Could you check a few things on this model? Use its own coordinates, in mm. Face numbers are marked on the shaded views. A direction names the side the tool comes from. Round coordinates to 2 decimals unless told otherwise and drop trailing zeros. Write each loop counter-clockwise with the first axis right and the second up, starting at its lowest first coordinate (ties: lowest second). Pieces come first, ordered by that corner, then holes. Notation, with made-up numbers: M -7,27.5 L 8,27.5 A19 ccw 8,38.5 Z; hole C -27.75,71.25 d10. An arc over 180 degrees is marked long. One line per item, written item: value. Start each with the question number.
(1) I want a section at B-B on z = 1. Please give me the cut outline in (x, y), and give its area (3 significant figures).
(2) I want a section at C-C on y = 0. Count the separate pieces of the cut face and the enclosed holes in it, and give its area (3 significant figures).
(3) I want a section at A-A on x = 0. Please give me the cut outline in (y, z) (3 decimals), and give its area (3 significant figures).
(4) I'm going to push flat-ended pins straight in: pin 1 Ø4 at (x, y) = (-7.874, 0) entering from +Z; pin 2 Ø1.5 at (y, z) = (3, 1) entering from -X; pin 3 Ø2 at (x, y) = (-9, 1.5) entering from +Z (3 decimals); pin 4 Ø4 at (x, z) = (8.5, 2) entering from +Y. Where does each tip first touch, or does it pass through?
(5) If I drill on L1, parallel to X at y = -2.75, z = 4.5; L2, parallel to X at y = 1, z = 3.25; L3, parallel to Y at x = 0, z = 2.9, over which ranges is the centre line in solid material (lowest first)?
(6) Which directions (+Z, -Z, +X, -X, +Y, -Y) give clear straight access to the entire face, cutting with the end or side of a thin tool? Please do the marked faces 1 and 2.
(7) Thinking about a two-plate mould opening in X: for the marked faces 3, 4 and 5, which applies, released by +X, released by -X, zero draft, split by the parting line, or undercut?
(8) I want a section at D-D on x = -6.5. Please give me the cut outline in (y, z) (3 decimals).
```python
from build123d import *

# Parameters (mm, degrees)
SKETCH1_R           = 3.302
SKETCH1_R_2         = 2.54
BOSS_EXTRUDE1_DEPTH = 3.81
SKETCH1_7_R         = 2.54
BOSS_EXTRUDE2_DEPTH = 3.81
SKETCH2_R           = 3.302
CUT_EXTRUDE1_DEPTH  = 0.635


with BuildPart() as part:
    # Sketch1 → Boss-Extrude1 (new body)
    with BuildSketch(Plane.XY):
        with BuildLine():
            Line((3.937, -3.81), (7.874, -3.81))
            ThreePointArc((7.874, -3.81), (11.684, 0), (7.874, 3.81))
            Line((7.874, 3.81), (3.937, 3.81))
            Line((3.937, 3.81), (3.937, 3.302))
            Line((3.937, 3.302), (4.92278669, 3.302))
            ThreePointArc((4.92278669, 3.302), (5.389414486, 2.994804631), (5.291688354, 2.44475))
            ThreePointArc((5.291688354, 2.44475), (4.318, 0), (5.291688354, -2.44475))
            ThreePointArc((5.291688354, -2.44475), (5.389414486, -2.994804631), (4.92278669, -3.302))
            Line((4.92278669, -3.302), (3.937, -3.302))
            Line((3.937, -3.302), (3.937, -3.81))
        make_face()
        with Locations((7.874, 0)):
            Circle(SKETCH1_R, mode=Mode.SUBTRACT)
        with Locations((7.874, 0)):
            Circle(SKETCH1_R)
        with Locations(Location((7.874, 0, 0), (0, 0, 180))):
            Circle(SKETCH1_R_2, mode=Mode.SUBTRACT)
    extrude(amount=BOSS_EXTRUDE1_DEPTH)


with BuildPart() as body_2:
    # Sketch1_7 → Boss-Extrude2 (new body)
    with BuildSketch(Plane.XY):
        with BuildLine():
            Line((3.937, -3.81), (3.937, -3.302))
            Line((3.937, -3.302), (2.95121331, -3.302))
            ThreePointArc((2.95121331, -3.302), (2.484585514, -2.994804631), (2.582311646, -2.44475))
            ThreePointArc((2.582311646, -2.44475), (3.556, 0), (2.582311646, 2.44475))
            ThreePointArc((2.582311646, 2.44475), (2.484585514, 2.994804631), (2.95121331, 3.302))
            Line((2.95121331, 3.302), (3.937, 3.302))
            Line((3.937, 3.302), (3.937, 3.81))
            Line((3.937, 3.81), (-3.937, 3.81))
            Line((-3.937, 3.81), (-3.937, 3.302))
            Line((-3.937, 3.302), (-2.95121331, 3.302))
            ThreePointArc((-2.95121331, 3.302), (-2.484585514, 2.994804631), (-2.582311646, 2.44475))
            ThreePointArc((-2.582311646, 2.44475), (-3.556, 0), (-2.582311646, -2.44475))
            ThreePointArc((-2.582311646, -2.44475), (-2.484585514, -2.994804631), (-2.95121331, -3.302))
            Line((-2.95121331, -3.302), (-3.937, -3.302))
            Line((-3.937, -3.302), (-3.937, -3.81))
            Line((-3.937, -3.81), (3.937, -3.81))
        make_face()
        with Locations(Location((0, 0, 0), (0, 0, 180))):
            Circle(SKETCH1_7_R, mode=Mode.SUBTRACT)
    extrude(amount=BOSS_EXTRUDE2_DEPTH)


with BuildPart() as cut_extrude1_tool:
    # Sketch2 → Cut-Extrude1 (new body)
    with BuildSketch(Plane.XY):
        with Locations((7.874, 0)):
            Circle(SKETCH2_R)
        Circle(SKETCH2_R)
    extrude(amount=CUT_EXTRUDE1_DEPTH)


with BuildPart() as part_1:
    add(part.part)

    # Cut-Extrude1: cut by cut_extrude1_tool
    add(cut_extrude1_tool.part, mode=Mode.SUBTRACT)


with BuildPart() as body_2_1:
    add(body_2.part)

    # Cut-Extrude1: cut by cut_extrude1_tool
    add(cut_extrude1_tool.part, mode=Mode.SUBTRACT)


with BuildPart() as body_3:
    # Mirror2: mirrored copy
    add(part_1.part.mirror(Plane(origin=(0, 0, 0), x_dir=(0, 0, 1), z_dir=(1, 0, 0))))


with BuildPart() as part_2:
    add(part_1.part)

    # Combine1: union body 3, body 2
    add(body_3.part)
    add(body_2_1.part)

    # Mirror3: part across plane


with BuildPart() as part_3:
    add(part_2.part)
    add(part_2.part.mirror(Plane.XY.offset(3.81)))


solid = part_3.part
```
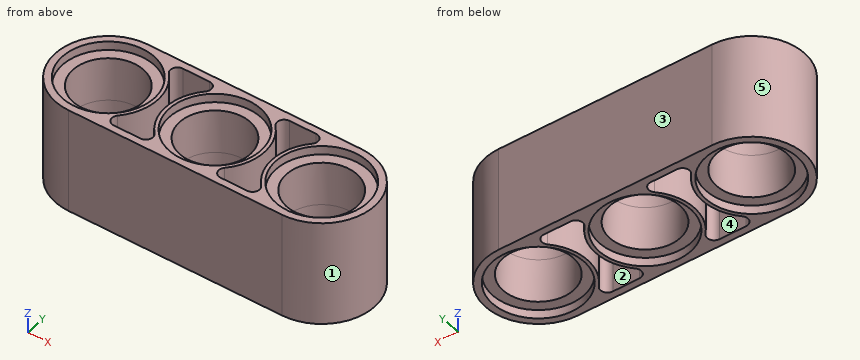
Found:
1. outline: M -7.87,-3.81 L 7.87,-3.81 A3.81 ccw 7.87,3.81 L -7.87,3.81 A3.81 ccw Z; hole C -7.87,0 d5.08; hole M -5.29,-2.44 A0.51 ccw -4.92,-3.3 L -2.95,-3.3 A0.51 ccw -2.58,-2.44 A3.56 cw -2.58,2.44 A0.51 ccw -2.95,3.3 L -4.92,3.3 A0.51 ccw -5.29,2.44 A3.56 cw Z; hole C 0,0 d5.08; hole M 2.58,-2.44 A0.51 ccw 2.95,-3.3 L 4.92,-3.3 A0.51 ccw 5.29,-2.44 A3.56 cw 5.29,2.44 A0.51 ccw 4.92,3.3 L 2.95,3.3 A0.51 ccw 2.58,2.44 A3.56 cw Z; hole C 7.87,0 d5.08
1. area: 81.7 mm²
2. separate pieces: 6
2. enclosed holes: 0
2. area: 44.5 mm²
3. outline: M -3.81,0 L -3.302,0 L -3.302,0.635 L -2.54,0.635 L -2.54,6.985 L -3.302,6.985 L -3.302,7.62 L -3.81,7.62 Z; M 2.54,0.635 L 3.302,0.635 L 3.302,0 L 3.81,0 L 3.81,7.62 L 3.302,7.62 L 3.302,6.985 L 2.54,6.985 Z
3. area: 17.4 mm²
4. pin 1: passes through
4. pin 2: stops at x = -10.95
4. pin 3: stops at z = 6.985
4. pin 4: stops at y = 3.81
5. L1: x = -10.51 to -5.43, -2.45 to 2.45, 5.43 to 10.51
5. L2: x = -11.55 to -10.21, -5.54 to -4.46, -3.41 to -2.33, 2.33 to 3.41, 4.46 to 5.54, 10.21 to 11.55
5. L3: y = -3.81 to -2.54, 2.54 to 3.81
6. face 1: +Z, -Z, +X
6. face 2: +Z, -Z
7. face 3: zero draft
7. face 4: undercut
7. face 5: released by -X
8. outline: M -3.81,0 L -3.003,0 L -3.003,0.635 L -2.136,0.635 L -2.136,6.985 L -3.003,6.985 L -3.003,7.62 L -3.81,7.62 Z; M 2.136,0.635 L 3.003,0.635 L 3.003,0 L 3.81,0 L 3.81,7.62 L 3.003,7.62 L 3.003,6.985 L 2.136,6.985 Z
